from build123d import *

# Parameters (mm, degrees)
SKETCH1_R               = 26
BOSS_EXTRUDE1_DEPTH     = 140
SKETCH2_W               = 200
SKETCH2_H               = 296
CUT_EXTRUDE1_DEPTH      = 126
CUT_EXTRUDE1_DEPTH_BACK = 126


with BuildPart() as part:
    # Sketch1 → Boss-Extrude1 (new body, symmetric)
    with BuildSketch(Plane.XY):
        with BuildLine():
            Line((125, 280), (-125, 280))
            Line((-125, 280), (-54.44483322, -13.105729116))
            ThreePointArc((-54.44483322, -13.105729116), (0, -56), (54.44483322, -13.105729116))
            Line((54.44483322, -13.105729116), (125, 280))
        make_face()
        Circle(SKETCH1_R, mode=Mode.SUBTRACT)
    extrude(amount=BOSS_EXTRUDE1_DEPTH, both=True)

    # Sketch2 → Cut-Extrude1 (cut, two sides)
    with BuildSketch(Plane(origin=(0, 0, 0), x_dir=(0, 0, -1), z_dir=(1, 0, 0))) as cut_extrude1_sk:
        with Locations((0, 92)):
            Rectangle(SKETCH2_W, SKETCH2_H)
    extrude(amount=CUT_EXTRUDE1_DEPTH, mode=Mode.SUBTRACT)
    extrude(cut_extrude1_sk.sketch, amount=-CUT_EXTRUDE1_DEPTH_BACK, mode=Mode.SUBTRACT)


solid = part.part
Verification items for the finished model (mm, model axes). A direction names the side the tool comes from. Coordinates: 2 decimals unless noted, no trailing zeros. Write each loop counter-clockwise with the first axis right and the second up, starting at its lowest first coordinate (ties: lowest second). Pieces come first, ordered by that corner, then holes. Notation, with made-up numbers: (-11.75, 1) -> (44.25, 1) arc R22 cw to (44.25, 31) -> close; hole circle Ø9 at (-35.75, 26.25). An arc over 180 degrees is marked (long way). One line per item, written item: value. Start each with the question number.
Q1. Cross-section at B-B on y = -21.5. Enter the section's corners in (x, z), and give its area (3 significant figures).
Q2. Go/stop test with a flat-tipped pin: P1, Ø10, axis at y = 35.5, z = 106, coming from the +X side. Record where the tip stops, or that it passes through.
Q3. Access from +Z, -Z, +X, -X, +Y, -Y to the whole of each face (thin tool, end or side, straight path). Record for faces 1 (the flat face through (2, 123, -100)), 2 (the flat face through (115.69, 241.32, -9.72)).
Q4. Cross-section at D-D on x = -104.5. Enter the section's corners in (y, z).
Q5. Mould release check, pull along Y, two halves, no side actions. Record for faces 3 (the cylindrical face through (-20.633, -15.821, 119.72)), 4 (the flat face through (2, 240, 1)), 5 (the flat face through (-2, 152, -140)): pulls with the +Y half, pulls with the -Y half, needs draft (parallel to the pull), parting line crosses it, or undercut.
Q6. Thickness scan on L1, parallel to Z at x = -4.5, y = 61; L2, parallel to Y at x = 0, z = 131; L3, parallel to Y at x = 95.5, z = -0.5. Record the ranges inside material, lowest first. Write a range as from..to.
Q7. Cross-section at A-A on x = 0. Enter the section's corners in (y, z).
Q8. Cross-section at C-C on y = 117. Enter the section's corners in (x, z), and give its area (3 significant figures).
Checked values:
1. outline: (-51.71, -140) -> (-14.62, -140) -> (-14.62, -100) -> (-51.71, -100) -> close; (-51.71, 100) -> (-14.62, 100) -> (-14.62, 140) -> (-51.71, 140) -> close; (14.62, -140) -> (51.71, -140) -> (51.71, -100) -> (14.62, -100) -> close; (14.62, 100) -> (51.71, 100) -> (51.71, 140) -> (14.62, 140) -> close
1. area: 5,930 mm²
2. P1: stops at x = 67.35
3. face 1: +X, -X, -Y
3. face 2: +Z, -Z, +X, -Y
4. outline: (194.84, -140) -> (280, -140) -> (280, 140) -> (194.84, 140) -> (194.84, 100) -> (240, 100) -> (240, -100) -> (194.84, -100) -> close
5. face 3: undercut
5. face 4: pulls with the -Y half
5. face 5: needs draft
6. L1: z = -140..-100, 100..140
6. L2: y = -56..-26, 26..280
6. L3: y = 240..280
7. outline: (-56, -140) -> (-26, -140) -> (-26, -100) -> (-56, -100) -> close; (-56, 100) -> (-26, 100) -> (-26, 140) -> (-56, 140) -> close; (26, -140) -> (280, -140) -> (280, 140) -> (26, 140) -> (26, 100) -> (240, 100) -> (240, -100) -> (26, -100) -> close
8. outline: (-85.76, -140) -> (85.76, -140) -> (85.76, -100) -> (-85.76, -100) -> close; (-85.76, 100) -> (85.76, 100) -> (85.76, 140) -> (-85.76, 140) -> close
8. area: 13,700 mm²
